Verification items for this drawing (mm, ordinates from the low corner). A direction names the side the tool comes from. Give positions to 0.01 mm unless a question says otherwise; leave off trailing zeros. Loops run counter-clockwise (first coordinate to the right, second up) from the corner with the lowest first, then second, coordinate; pieces in that order, holes last. Notation, with made-up numbers: M 77,-2.75 L 122,-2.75 A12 ccw 122,6.25 Z; hole C -13.5,-10 d2. An arc over 180 degrees is marked long. Use a Markdown table: item, result.
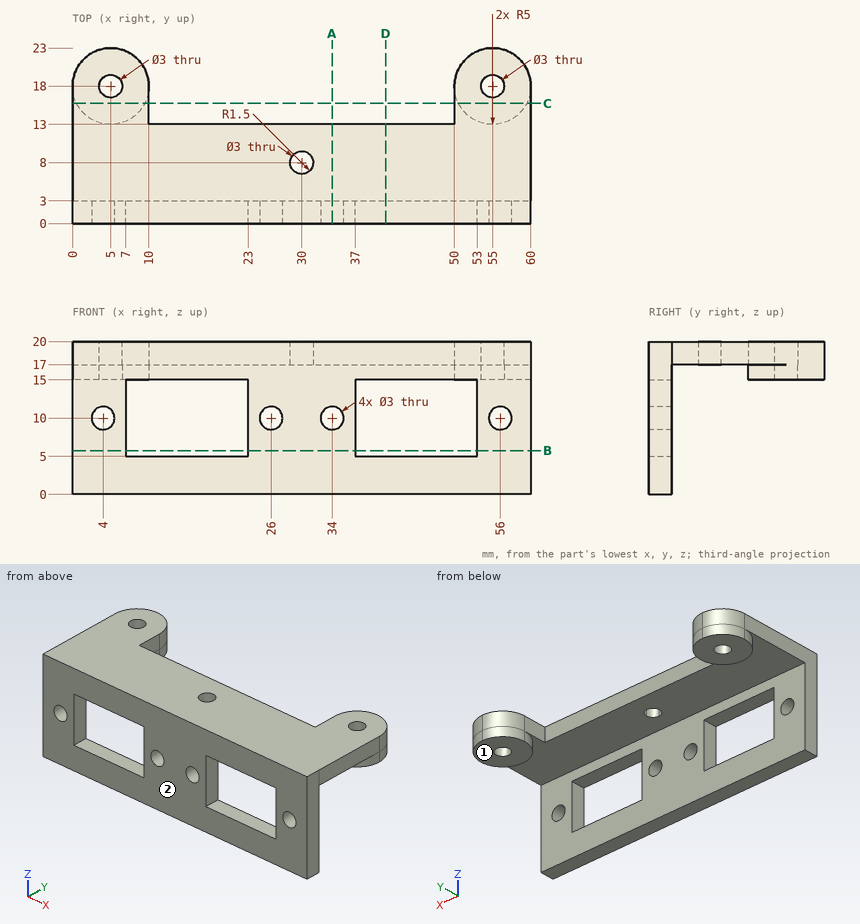
(1) Set-up check for the marked faces 1 and 2: record each of +Z, -Z, +X, -X, +Y, -Y from which the full face is reachable in a straight line by a thin tool's end or side.
Results below:
| item | result |
|---|---|
| face 1 | -Z, +X, -X, +Y |
| face 2 | +Z, -Z, +X, -X, -Y |
(2) Cross-section at D-D on x = 41. Record the cut outline in (y, z).
Results below:
| item | result |
|---|---|
| outline | M 0,0 L 3,0 L 3,5 L 0,5 Z; M 0,15 L 3,15 L 3,17 L 13,17 L 13,20 L 0,20 Z |
(3) Cross-section at B-B on z = 5.75. Record the cut outline in (x, y), then the cut area to 3 significant figures.
Results below:
| item | result |
|---|---|
| outline | M 0,0 L 7,0 L 7,3 L 0,3 Z; M 23,0 L 37,0 L 37,3 L 23,3 Z; M 53,0 L 60,0 L 60,3 L 53,3 Z |
| area | 84.0 mm^2 |
(4) Cross-section at C-C on y = 15.75. Record the cut outline in (x, z).
Results below:
| item | result |
|---|---|
| outline | M 0,17 L 0.53,17 L 0.53,15 L 9.47,15 L 9.47,17 L 10,17 L 10,20 L 0,20 Z; M 50,17 L 50.53,17 L 50.53,15 L 59.47,15 L 59.47,17 L 60,17 L 60,20 L 50,20 Z |
(5) Gauge pin test, flat ends, axial feed: P1, Ø1.8, axis at x = 5, y = 18, coming from the +Z side; P2, Ø5, axis at x = 44, y = 6.5, coming from the -Z side; P3, Ø0.9, axis at x = 34, z = 18.5, coming from the +Y side; P4, Ø3.5, axis at x = 55, y = 18, coming from the -Z side. Record the tip position at first contact, or that the pin passes through.
Results below:
| item | result |
|---|---|
| P1 | through |
| P2 | z = 17 |
| P3 | y = 13 |
| P4 | z = 15 |
(6) Cross-section at A-A on x = 34. Record the cut outline in (y, z), then the cut area to 3 significant figures.
Results below:
| item | result |
|---|---|
| outline | M 0,0 L 3,0 L 3,8.5 L 0,8.5 Z; M 0,11.5 L 3,11.5 L 3,17 L 13,17 L 13,20 L 0,20 Z |
| area | 81.0 mm^2 |
(7) Material ranges on line 1 (Z direction, x = 26, y = 1.9); line 2 (X direction, y = 15, z = 18.5); line 3 (Y direction, x = 53.5, z = 4.5), recorded low to high.
Results below:
| item | result |
|---|---|
| line 1 | 0 to 8.5, 11.5 to 20 |
| line 2 | 0 to 10, 50 to 60 |
| line 3 | 0 to 3 |
